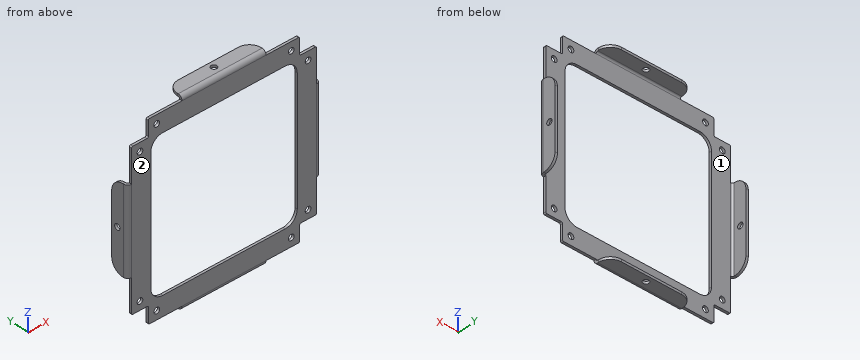
```python
from build123d import *

# Parameters (mm, degrees)
SKETCH1_W          = 77
SKETCH1_H          = 77
BASE_FLANGE1_DEPTH = 1
EDGE_FLANGE1_DEPTH = 35
EDGE_FLANGE2_DEPTH = 35
EDGE_FLANGE3_DEPTH = 35
EDGE_FLANGE4_DEPTH = 35
CUT_EXTRUDE1_DEPTH = 58.218598018
FILLET1_R          = 0.5
FILLET2_R          = 5
M2_HOLE1_AA_D      = 2.4
M2_HOLE2_AB_D      = 2.4
M2_HOLE3_AC_D      = 2.4


# Sheet-metal steps are written as plain solids
with BuildPart() as part:
    # Sketch1 → Base-Flange1 (new body)
    with BuildSketch(Plane(origin=(0, 0, 0), x_dir=(1, 0, 0), z_dir=(0, 1, 0))):
        Rectangle(SKETCH1_W, SKETCH1_H)
    extrude(amount=-BASE_FLANGE1_DEPTH)

    # Edge-Flange1 section (across the edge) → Edge-Flange1 (add)
    with BuildSketch(Plane(origin=(-17.5, 0, 39.2366), x_dir=(0, 0, -1), z_dir=(1, 0, 0))):
        with BuildLine():
            Line((-1, 0.7366), (-1, 6))
            Line((-1, 6), (0, 6))
            Line((0, 6), (0, 0.7366))
            ThreePointArc((0, 0.7366), (0.215745145, 0.215745145), (0.7366, 0))
            Line((0.7366, 0), (0.7366, -1))
            ThreePointArc((0.7366, -1), (-0.491361636, -0.491361636), (-1, 0.7366))
        make_face()
    extrude(amount=EDGE_FLANGE1_DEPTH)

    # Edge-Flange2 section (across the edge) → Edge-Flange2 (add)
    with BuildSketch(Plane(origin=(17.5, 0, -39.2366), x_dir=(0, 0, 1), z_dir=(-1, 0, 0))):
        with BuildLine():
            Line((-1, 0.7366), (-1, 6))
            Line((-1, 6), (0, 6))
            Line((0, 6), (0, 0.7366))
            ThreePointArc((0, 0.7366), (0.215745145, 0.215745145), (0.7366, 0))
            Line((0.7366, 0), (0.7366, -1))
            ThreePointArc((0.7366, -1), (-0.491361636, -0.491361636), (-1, 0.7366))
        make_face()
    extrude(amount=EDGE_FLANGE2_DEPTH)

    # Edge-Flange3 section (across the edge) → Edge-Flange3 (add)
    with BuildSketch(Plane(origin=(-39.2366, 0, -17.5), x_dir=(1, 0, 0), z_dir=(0, 0, 1))):
        with BuildLine():
            Line((-1, 0.7366), (-1, 6))
            Line((-1, 6), (0, 6))
            Line((0, 6), (0, 0.7366))
            ThreePointArc((0, 0.7366), (0.215745145, 0.215745145), (0.7366, 0))
            Line((0.7366, 0), (0.7366, -1))
            ThreePointArc((0.7366, -1), (-0.491361636, -0.491361636), (-1, 0.7366))
        make_face()
    extrude(amount=EDGE_FLANGE3_DEPTH)

    # Edge-Flange4 section (across the edge) → Edge-Flange4 (add)
    with BuildSketch(Plane(origin=(39.2366, 0, 17.5), x_dir=(-1, 0, 0), z_dir=(0, 0, -1))):
        with BuildLine():
            Line((-1, 0.7366), (-1, 6))
            Line((-1, 6), (0, 6))
            Line((0, 6), (0, 0.7366))
            ThreePointArc((0, 0.7366), (0.215745145, 0.215745145), (0.7366, 0))
            Line((0.7366, 0), (0.7366, -1))
            ThreePointArc((0.7366, -1), (-0.491361636, -0.491361636), (-1, 0.7366))
        make_face()
    extrude(amount=EDGE_FLANGE4_DEPTH)

    # Sketch18 → Cut-Extrude1 (cut, through all)
    with BuildSketch(Plane(origin=(0, 0, 0), x_dir=(1, 0, 0), z_dir=(0, 1, 0))):
        with BuildLine():
            Line((-25.5, -30.5), (25.5, -30.5))
            ThreePointArc((25.5, -30.5), (29.035533906, -29.035533906), (30.5, -25.5))
            Line((30.5, -25.5), (30.5, 25.5))
            ThreePointArc((30.5, 25.5), (29.035533906, 29.035533906), (25.5, 30.5))
            Line((25.5, 30.5), (-25.5, 30.5))
            ThreePointArc((-25.5, 30.5), (-29.035533906, 29.035533906), (-30.5, 25.5))
            Line((-30.5, 25.5), (-30.5, -25.5))
            ThreePointArc((-30.5, -25.5), (-29.035533906, -29.035533906), (-25.5, -30.5))
        make_face()
        with BuildLine():
            Line((-38.5, 38.5), (-31.5, 38.5))
            Line((-31.5, 38.5), (-31.5, 32))
            ThreePointArc((-31.5, 32), (-31.646446609, 31.646446609), (-32, 31.5))
            Line((-32, 31.5), (-38.5, 31.5))
            Line((-38.5, 31.5), (-38.5, 38.5))
        make_face()
        with BuildLine():
            Line((38.5, 38.5), (31.5, 38.5))
            Line((31.5, 38.5), (31.5, 32))
            ThreePointArc((31.5, 32), (31.646446609, 31.646446609), (32, 31.5))
            Line((32, 31.5), (38.5, 31.5))
            Line((38.5, 31.5), (38.5, 38.5))
        make_face()
        with BuildLine():
            Line((38.5, -38.5), (31.5, -38.5))
            Line((31.5, -38.5), (31.5, -32))
            ThreePointArc((31.5, -32), (31.646446609, -31.646446609), (32, -31.5))
            Line((32, -31.5), (38.5, -31.5))
            Line((38.5, -31.5), (38.5, -38.5))
        make_face()
        with BuildLine():
            Line((-38.5, -38.5), (-31.5, -38.5))
            Line((-31.5, -38.5), (-31.5, -32))
            ThreePointArc((-31.5, -32), (-31.646446609, -31.646446609), (-32, -31.5))
            Line((-32, -31.5), (-38.5, -31.5))
            Line((-38.5, -31.5), (-38.5, -38.5))
        make_face()
    extrude(amount=-CUT_EXTRUDE1_DEPTH, mode=Mode.SUBTRACT)

    # Fillet1
    fillet1_edges = [part.edges().sort_by_distance(p)[0] for p in [
        (31.5, -0.5, -38.5),
        (38.5, -0.5, -31.5),
        (38.5, -0.5, 31.5),
        (31.5, -0.5, 38.5),
        (-31.5, -0.5, 38.5),
        (-38.5, -0.5, 31.5),
        (-38.5, -0.5, -31.5),
        (-31.5, -0.5, -38.5),
    ]]
    fillet(fillet1_edges, radius=FILLET1_R)

    # Fillet2
    fillet2_edges = [part.edges().sort_by_distance(p)[0] for p in [
        (39.7366, 6, 17.5),
        (39.7366, 6, -17.5),
        (-17.5, 6, 39.7366),
        (17.5, 6, 39.7366),
        (17.5, 6, -39.7366),
        (-17.5, 6, -39.7366),
        (-39.7366, 6, -17.5),
        (-39.7366, 6, 17.5),
    ]]
    fillet(fillet2_edges, radius=FILLET2_R)

    # M2 Hole1 - AA (through all)
    with Locations(Plane(origin=(-35, 0, -28), x_dir=(0, 0, 1), z_dir=(0, 1, 0))):
        with Locations((0, 0), (-7, 7), (-7, 63), (0, 70), (56, 0), (63, 7), (63, 63), (56, 70)):
            Hole(M2_HOLE1_AA_D / 2)

    # M2 Hole2 - AB (through all)
    with Locations(Plane.ZY.offset(40.2366)):
        with Locations((0, 3.5)):
            Hole(M2_HOLE2_AB_D / 2)

    # M2 Hole3 - AC (through all)
    with Locations(Plane.XY.offset(40.2366)):
        with Locations((0, 3.5)):
            Hole(M2_HOLE3_AC_D / 2)


solid = part.part
```
The listing builds one solid part. Answer for the finished solid, in the listing's coordinates (mm). Face numbers are marked on the shaded views. Coordinates: 2 decimals unless noted, no trailing zeros. Loops run counter-clockwise (first coordinate to the right, second up) from the corner with the lowest first, then second, coordinate; pieces in that order, holes last. Notation, with made-up numbers: (26.5, 0) -> (40.5, 0) arc R31 cw to (40.5, 37) -> close; hole circle Ø6 at (74, 46). An arc over 180 degrees is marked (long way). Return JSON: item names as keys, results as strings. Group by question number.
(1) A cutting plane is placed at D-D on x = 0. Write down the section's boundary in (y, z).
(2) A cutting plane is placed at A-A on z = -35. Write down the section's boundary in (x, y), and give its area (3 significant figures).
(3) Given pin 1 Ø0.9 at (y, z) = (0, -39.5) entering from +X; pin 2 Ø1.1 at (y, z) = (-0.5, -23.5) entering from +X; pin 3 Ø1.1 at (y, z) = (-0.5, -25.5) entering from -X; pin 4 Ø1 at (x, y) = (-26, 1.5) entering from -Z, each flat-ended and moving along its own axis, determine where each tip first touches the part or whether it passes through.
(4) Determine the mould class of the marked faces 1 and 2 for opening direction X: released by +X, released by -X, zero draft, split by the parting line, or undercut.
(5) A cutting plane is placed at B-B on x = -20. Write down the section's boundary in (y, z), and give its area (3 significant figures).
(6) A cutting plane is placed at C-C on z = -3. Write down the section's boundary in (x, y), and give its area (3 significant figures).
(7) Find the intervals of material crossed by probe 1 along X at (y, z) = (-0.65, 35); probe 2 along X at (y, z) = (1, -15), in increasing order. Write a range as from..to.
The answers:
{
 "1": {"outline": "(-1, -38.5) arc R1.74 ccw to (0.74, -40.24) -> (2.3, -40.24) -> (2.3, -39.24) -> (0.74, -39.24) arc R0.74 cw to (0, -38.5) -> (0, -30.5) -> (-1, -30.5) -> close; (-1, 30.5) -> (0, 30.5) -> (0, 38.5) arc R0.74 cw to (0.74, 39.24) -> (2.3, 39.24) -> (2.3, 40.24) -> (0.74, 40.24) arc R1.74 ccw to (-1, 38.5) -> close; (4.7, -40.24) -> (6, -40.24) -> (6, -39.24) -> (4.7, -39.24) -> close; (4.7, 39.24) -> (6, 39.24) -> (6, 40.24) -> (4.7, 40.24) -> close"},
 "2": {"outline": "(-31.5, -1) -> (-29.2, -1) -> (-29.2, 0) -> (-31.5, 0) -> close; (-26.8, -1) -> (26.8, -1) -> (26.8, 0) -> (-26.8, 0) -> close; (29.2, -1) -> (31.5, -1) -> (31.5, 0) -> (29.2, 0) -> close", "area": "58.2 mm^2"},
 "3": {"pin 1": "stops at x = 17.5", "pin 2": "stops at x = 38.5", "pin 3": "stops at x = -38.5", "pin 4": "passes through"},
 "4": {"face 1": "undercut", "face 2": "zero draft"},
 "5": {"outline": "(-1, -38.5) -> (0, -38.5) -> (0, -30.5) -> (-1, -30.5) -> close; (-1, 30.5) -> (0, 30.5) -> (0, 38.5) -> (-1, 38.5) -> close", "area": "16.0 mm^2"},
 "6": {"outline": "(-40.24, 0.74) arc R1.74 ccw to (-38.5, -1) -> (-30.5, -1) -> (-30.5, 0) -> (-38.5, 0) arc R0.74 cw to (-39.24, 0.74) -> (-39.24, 6) -> (-40.24, 6) -> close; (30.5, -1) -> (38.5, -1) arc R1.74 ccw to (40.24, 0.74) -> (40.24, 6) -> (39.24, 6) -> (39.24, 0.74) arc R0.74 cw to (38.5, 0) -> (30.5, 0) -> close", "area": "30.4 mm^2"},
 "7": {"probe 1": "x = -31.5..-29.2, -26.8..26.8, 29.2..31.5", "probe 2": "x = -40.24..-39.24, 39.24..40.24"}
}
